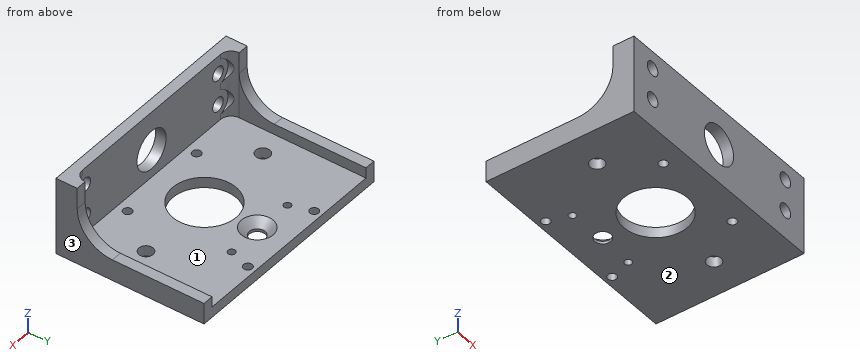
from build123d import *

# Parameters (mm, degrees)
SKETCH1_W                                            = 64
SKETCH1_H                                            = 39
SKETCH1_R                                            = 9
BOSS_EXTRUDE1_DEPTH                                  = 3
SKETCH2_W                                            = 3
SKETCH2_H                                            = 39
BOSS_EXTRUDE2_DEPTH                                  = 3
SKETCH3_W                                            = 64
SKETCH3_H                                            = 22
BOSS_EXTRUDE3_DEPTH                                  = 3
SKETCH4_W                                            = 3
SKETCH4_H                                            = 16
BOSS_EXTRUDE4_DEPTH                                  = 3
FILLET1_R                                            = 10
F_4_0_4_DIAMETER_HOLE1_D                             = 4
F_4_0_4_DIAMETER_HOLE1_DEPTH                         = 15
F_4_0_4_DIAMETER_HOLE1_TIP                           = 1.201721238
CSK_FOR_M4_HEX_SOCKET_COUNTERSUNK_CAP_SC_D           = 4.5
CSK_FOR_M4_HEX_SOCKET_COUNTERSUNK_CAP_SC_DEPTH       = 10
CSK_FOR_M4_HEX_SOCKET_COUNTERSUNK_CAP_SC_CSINK_D     = 8.96
CSK_FOR_M4_HEX_SOCKET_COUNTERSUNK_CAP_SC_CSINK_ANGLE = 90
CSK_FOR_M4_HEX_SOCKET_COUNTERSUNK_CAP_SC_TIP         = 1.351936393
M2_5_TAPPED_HOLE1_D                                  = 2.05
M2_5_TAPPED_HOLE1_DEPTH                              = 7.25
M2_5_TAPPED_HOLE1_TIP                                = 0.615882135
M3_TAPPED_HOLE1_D                                    = 2.5
M3_TAPPED_HOLE1_DEPTH                                = 8.5
M3_TAPPED_HOLE1_TIP                                  = 0.751075774
FILLET4_R                                            = 3
SKETCH19_R                                           = 2
CUT_EXTRUDE1_DEPTH                                   = 10
SKETCH20_R                                           = 5.5
CUT_EXTRUDE2_DEPTH                                   = 10
SKETCH21_R                                           = 3.75
CUT_EXTRUDE3_DEPTH                                   = 10


with BuildPart() as part:
    # Sketch1 → Boss-Extrude1 (new body)
    with BuildSketch(Plane.XY):
        with Locations((0, 4.5)):
            Rectangle(SKETCH1_W, SKETCH1_H)
        Circle(SKETCH1_R, mode=Mode.SUBTRACT)
    extrude(amount=BOSS_EXTRUDE1_DEPTH)

    # Sketch2 → Boss-Extrude2 (add)
    with BuildSketch(Plane.XY.offset(3)):
        with Locations((-30.5, 4.5)):
            Rectangle(SKETCH2_W, SKETCH2_H)
        with Locations((30.5, 4.5)):
            Rectangle(SKETCH2_W, SKETCH2_H)
    extrude(amount=BOSS_EXTRUDE2_DEPTH)

    # Sketch3 → Boss-Extrude3 (add)
    with BuildSketch(Plane.XZ.offset(15)):
        with Locations((0, 11)):
            Rectangle(SKETCH3_W, SKETCH3_H)
    extrude(amount=BOSS_EXTRUDE3_DEPTH)

    # Sketch4 → Boss-Extrude4 (add)
    with BuildSketch(Plane(origin=(0, -15, 0), x_dir=(1, 0, 0), z_dir=(0, 1, 0))):
        with Locations((-30.5, -14)):
            Rectangle(SKETCH4_W, SKETCH4_H)
        with Locations((30.5, -14)):
            Rectangle(SKETCH4_W, SKETCH4_H)
    extrude(amount=BOSS_EXTRUDE4_DEPTH)

    # Fillet1
    fillet1_edges = [part.edges().sort_by_distance(p)[0] for p in [
        (-30.5, -12, 6),
        (30.5, -12, 6),
    ]]
    fillet(fillet1_edges, radius=FILLET1_R)

    # Ø4.0 (4) Diameter Hole1
    with Locations(Plane(origin=(0, 0, 0), x_dir=(-1, 0, 0), z_dir=(0, 0, -1))):
        with Locations((-22, 0), (22, 0)):
            Hole(F_4_0_4_DIAMETER_HOLE1_D / 2, depth=F_4_0_4_DIAMETER_HOLE1_DEPTH)
            with Locations((0, 0, -(F_4_0_4_DIAMETER_HOLE1_DEPTH + F_4_0_4_DIAMETER_HOLE1_TIP / 2))):  # 118° drill point
                Cone(0, F_4_0_4_DIAMETER_HOLE1_D / 2, F_4_0_4_DIAMETER_HOLE1_TIP, mode=Mode.SUBTRACT)

    # CSK for M4 Hex Socket Countersunk Cap Screw1
    with Locations(Plane.XY.offset(3)):
        with Locations((0, 15)):
            CounterSinkHole(CSK_FOR_M4_HEX_SOCKET_COUNTERSUNK_CAP_SC_D / 2, CSK_FOR_M4_HEX_SOCKET_COUNTERSUNK_CAP_SC_CSINK_D / 2, depth=CSK_FOR_M4_HEX_SOCKET_COUNTERSUNK_CAP_SC_DEPTH, counter_sink_angle=CSK_FOR_M4_HEX_SOCKET_COUNTERSUNK_CAP_SC_CSINK_ANGLE)
            with Locations((0, 0, -(CSK_FOR_M4_HEX_SOCKET_COUNTERSUNK_CAP_SC_DEPTH + CSK_FOR_M4_HEX_SOCKET_COUNTERSUNK_CAP_SC_TIP / 2))):  # 118° drill point
                Cone(0, CSK_FOR_M4_HEX_SOCKET_COUNTERSUNK_CAP_SC_D / 2, CSK_FOR_M4_HEX_SOCKET_COUNTERSUNK_CAP_SC_TIP, mode=Mode.SUBTRACT)

    # M2.5 Tapped Hole1
    with Locations(Plane.XY.offset(3)):
        with Locations((-10.5, 15.66), (10.5, 15.66)):
            Hole(M2_5_TAPPED_HOLE1_D / 2, depth=M2_5_TAPPED_HOLE1_DEPTH)
            with Locations((0, 0, -(M2_5_TAPPED_HOLE1_DEPTH + M2_5_TAPPED_HOLE1_TIP / 2))):  # 118° drill point
                Cone(0, M2_5_TAPPED_HOLE1_D / 2, M2_5_TAPPED_HOLE1_TIP, mode=Mode.SUBTRACT)

    # M3 Tapped Hole1
    with Locations(Plane.XY.offset(3)):
        with Locations((-12.5, 21.75), (12.5, 21.75), (13, -12), (-13, -12)):
            Hole(M3_TAPPED_HOLE1_D / 2, depth=M3_TAPPED_HOLE1_DEPTH)
            with Locations((0, 0, -(M3_TAPPED_HOLE1_DEPTH + M3_TAPPED_HOLE1_TIP / 2))):  # 118° drill point
                Cone(0, M3_TAPPED_HOLE1_D / 2, M3_TAPPED_HOLE1_TIP, mode=Mode.SUBTRACT)

    # Fillet4
    fillet4_edges = [part.edges().sort_by_distance(p)[0] for p in [
        (29, -15, 12.5),
        (-29, -15, 12.5),
    ]]
    fillet(fillet4_edges, radius=FILLET4_R - 0.0001)  # a hair under: the kernel refuses the full size

    # Sketch19 → Cut-Extrude1 (cut)
    with BuildSketch(Plane.XZ.offset(18)):
        with Locations(Location((-25, 8, 0), (0, 0, 270))):
            Circle(SKETCH19_R)
        with Locations(Location((25, 8, 0), (0, 0, 270))):
            Circle(SKETCH19_R)
        with Locations(Location((-25, 17, 0), (0, 0, 270))):
            Circle(SKETCH19_R)
        with Locations(Location((25, 17, 0), (0, 0, 270))):
            Circle(SKETCH19_R)
    extrude(amount=-CUT_EXTRUDE1_DEPTH, mode=Mode.SUBTRACT)

    # Sketch20 → Cut-Extrude2 (cut)
    with BuildSketch(Plane(origin=(0, -15, 0), x_dir=(1, 0, 0), z_dir=(0, 1, 0))):
        with Locations(Location((0, -11, 0), (0, 0, 270))):
            Circle(SKETCH20_R)
    extrude(amount=-CUT_EXTRUDE2_DEPTH, mode=Mode.SUBTRACT)

    # Sketch21 → Cut-Extrude3 (cut)
    with BuildSketch(Plane(origin=(0, -15, 0), x_dir=(1, 0, 0), z_dir=(0, 1, 0))):
        with Locations((-25, -8)):
            Circle(SKETCH21_R)
        with Locations((-25, -17)):
            Circle(SKETCH21_R)
        with Locations((25, -8)):
            Circle(SKETCH21_R)
        with Locations((25, -17)):
            Circle(SKETCH21_R)
    extrude(amount=CUT_EXTRUDE3_DEPTH, mode=Mode.SUBTRACT)


solid = part.part
Work out the finished part from the listing and answer in its coordinate system (mm). Face numbers are marked on the shaded views. Give positions to 0.01 mm unless a question says otherwise; leave off trailing zeros. Order: outer loops, then holes, each group sorted by start corner. A loop starts at its lowest first (then second) coordinate and runs counter-clockwise, first axis right, second up. Notation, with made-up numbers: (47.5, 28.5) -> (82.5, 28.5) arc R6 cw to (82.5, 34.5) -> close; hole circle Ø4 at (10.25, 12.25). An arc over 180 degrees is marked (long way). One line per item, written item: value.
Item 1: Find section D-D, the plane z = 18.25. State how many separate pieces and enclosed holes the cut face has, plus the area to 3 significant figures.
Answer sheet:
separate pieces: 3
enclosed holes: 0
area: 193 mm²
Item 2: Determine the mould class of the marked faces 1, 2 and 3 for opening direction X: released by +X, released by -X, zero draft, split by the parting line, or undercut.
Answer sheet:
face 1: undercut
face 2: zero draft
face 3: released by +X
Item 3: Find section B-B, the plane y = 21.75. Give the vertices of the cut face in (x, z).
Answer sheet:
outline: (-32, 0) -> (-13.75, 0) -> (-13.75, 3) -> (-29, 3) -> (-29, 6) -> (-32, 6) -> close; (-11.25, 0) -> (11.25, 0) -> (11.25, 3) -> (-11.25, 3) -> close; (13.75, 0) -> (32, 0) -> (32, 6) -> (29, 6) -> (29, 3) -> (13.75, 3) -> close
Item 4: Straight lines are drawn through the part: probe 1 along X at (y, z) = (15, 0.6); probe 2 along Y at (x, z) = (-10.5, 0.8) (3 decimals). For each, find the intervals that lie inside material, in ascending order.
Answer sheet:
probe 1: -32 to -11.28, -9.72 to -2.25, 2.25 to 9.72, 11.28 to 32
probe 2: -18 to 14.635, 16.685 to 24
Item 5: Find section A-A, the plane x = -10.5. Give the vertices of the cut face in (y, z) (3 decimals), plus the area to 3 significant figures.
Answer sheet:
outline: (-18, 0) -> (14.635, 0) -> (14.635, 3) -> (-15, 3) -> (-15, 22) -> (-18, 22) -> close; (16.685, 0) -> (24, 0) -> (24, 3) -> (16.685, 3) -> close
area: 177 mm²
Item 6: Flat-ended cylindrical pins translate along their axes: P1, Ø8, axis at x = -6.5, z = 14.5, coming from the +Y side; P2, Ø11.5, axis at x = 13.5, y = 4.5, coming from the +Z side; P3, Ø14.5, axis at x = 0, y = 0, coming from the +Z side; P4, Ø2.5, axis at x = -30, y = 10.5, coming from the +Z side. Find the tip coordinate at first contact, or state that the pin passes through.
Answer sheet:
P1: y = -15
P2: z = 3
P3: through
P4: z = 6
Item 7: Find section C-C, the plane y = -3. Give the vertices of the cut face in (x, z).
Answer sheet:
outline: (-32, 0) -> (-8.49, 0) -> (-8.49, 3) -> (-29, 3) -> (-29, 6.05) -> (-32, 6.05) -> close; (8.49, 0) -> (32, 0) -> (32, 6.05) -> (29, 6.05) -> (29, 3) -> (8.49, 3) -> close
